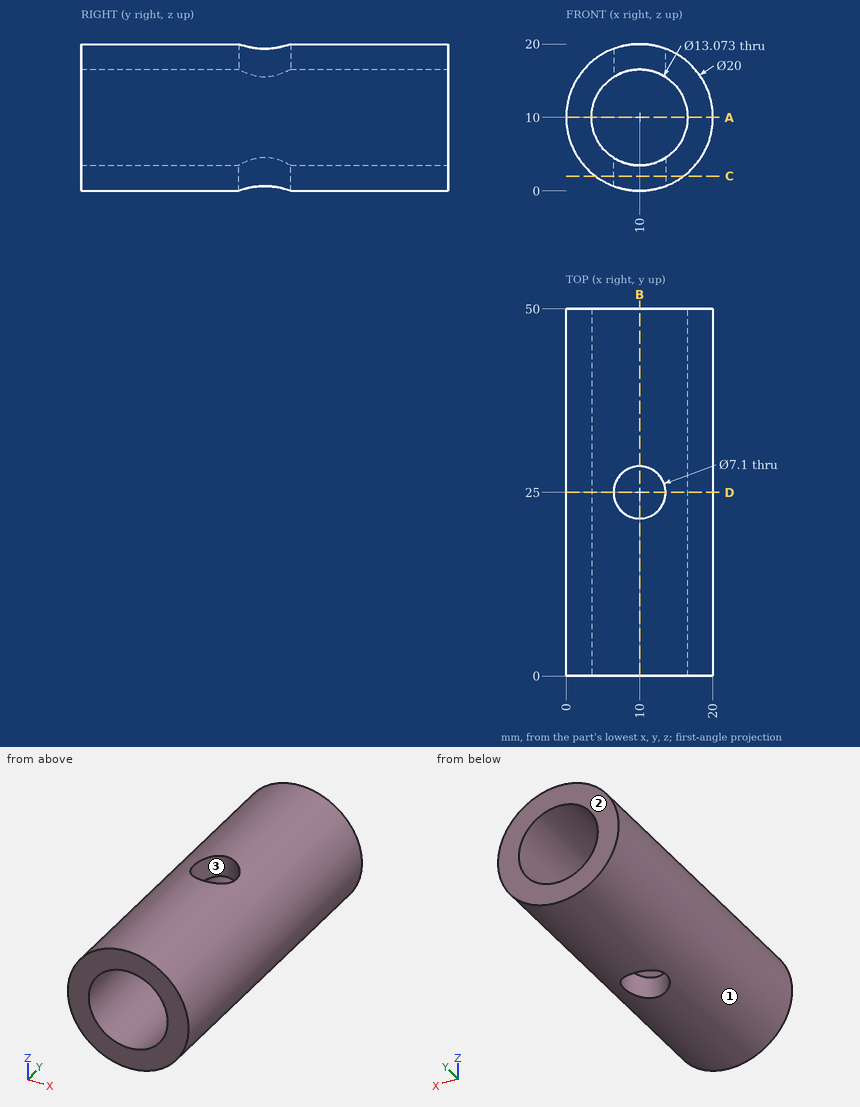
Source: three-view drawing plus pictorial views. Frame: mm from the lowest corner of the part. Coordinates: 2 decimals unless noted, no trailing zeros. Order: outer loops, then holes, each group sorted by start corner. A loop starts at its lowest first (then second) coordinate and runs counter-clockwise, first axis right, second up.
Item 1: Pull-direction query (X, two-part tool) for the marked faces 1, 2 and 3; classes: pulls with the +X half, pulls with the -X half, needs draft (parallel to the pull), parting line crosses it, or undercut.
Output values:
face 1: parting line crosses it
face 2: needs draft
face 3: undercut
Item 2: Cut plane D-D (y = 25). Return loops of the section in (x, z), plus the area to 3 significant figures.
Output values:
outline: (6.45, 0.65) - (6.45, 4.51) arc R6.54 cw to (6.45, 15.49) - (6.45, 19.35) arc R10 ccw to start; (13.55, 0.65) arc R10 ccw to (13.55, 19.35) - (13.55, 15.49) arc R6.54 cw to (13.55, 4.51) - close
area: 129 mm2
Item 3: Material intervals for line 1 (Z direction, x = 10, y = 37.5); line 2 (Y direction, x = 10, z = 17.6); line 3 (X direction, y = 12, z = 10.25), sorted ascending.
Output values:
line 1: z = 0 to 3.46, 16.54 to 20
line 2: y = 0 to 21.45, 28.55 to 50
line 3: x = 0 to 3.47, 16.53 to 20
Item 4: First-contact query: P1, Ø5, axis at y = 14.5, z = 5, coming from the -X side; P2, Ø8, axis at x = 10, z = 10, coming from the -Y side; P3, Ø4, axis at x = 3.5, y = 20, coming from the -Z side; P4, Ø4, axis at y = 44.5, z = 17, coming from the +X side. Flat tips, straight axial feed; report the tip coordinate or a pass-through.
Output values:
P1: stops at x = 0.32
P2: passes through
P3: stops at z = 1.07
P4: stops at x = 18.66
Item 5: Cut plane C-C (z = 2). Return loops of the section in (x, y).
Output values:
outline: (4, 0) - (16, 0) - (16, 50) - (4, 50) - close; hole circle Ø7.1 at (10, 25)
Item 6: Cut plane A-A (z = 10). Return loops of the section in (x, y).
Output values:
outline: (0, 0) - (3.46, 0) - (3.46, 50) - (0, 50) - close; (16.54, 0) - (20, 0) - (20, 50) - (16.54, 50) - close
Item 7: Cut plane B-B (x = 10). Return loops of the section in (y, z).
Output values:
outline: (0, 0) - (21.45, 0) - (21.45, 3.46) - (0, 3.46) - close; (0, 16.54) - (21.45, 16.54) - (21.45, 20) - (0, 20) - close; (28.55, 0) - (50, 0) - (50, 3.46) - (28.55, 3.46) - close; (28.55, 16.54) - (50, 16.54) - (50, 20) - (28.55, 20) - close
